```python
from build123d import *

# Parameters (mm, degrees)
SKETCH1_R           = 1.5
SKETCH1_R_2         = 1.375
SKETCH1_R_3         = 1.6
SKETCH1_R_4         = 1.625
SKETCH1_R_5         = 3.5687
SKETCH1_W           = 50
SKETCH1_H           = 41.5
BOSS_EXTRUDE1_DEPTH = 12.7


with BuildPart() as part:
    # Sketch1 → Boss-Extrude1 (new body)
    with BuildSketch(Plane(origin=(0, 0, 0), x_dir=(1, 0, 0), z_dir=(0, 1, 0))):
        with BuildLine():
            Line((175, -200), (175, 200))
            ThreePointArc((175, 200), (0, 265.753645318), (-175, 200))
            Line((-175, 200), (-175, -200))
            ThreePointArc((-175, -200), (-105.083237909, -244.095295142), (-25, -264.575131106))
            ThreePointArc((-25, -264.575131106), (-12.51388125, -265.458853264), (0, -265.753645318))
            ThreePointArc((0, -265.753645318), (12.51388125, -265.458853264), (25, -264.575131106))
            ThreePointArc((25, -264.575131106), (105.083237909, -244.095295142), (175, -200))
        make_face()
        with Locations((-31, -219.575131106)):
            Circle(SKETCH1_R, mode=Mode.SUBTRACT)
        with Locations((31, -219.575131106)):
            Circle(SKETCH1_R, mode=Mode.SUBTRACT)
        with Locations((22.5, -166)):
            Circle(SKETCH1_R_2, mode=Mode.SUBTRACT)
        with Locations((-31, -254.575131106)):
            Circle(SKETCH1_R, mode=Mode.SUBTRACT)
        with Locations((31, -254.575131106)):
            Circle(SKETCH1_R, mode=Mode.SUBTRACT)
        with Locations((-35.5, -166)):
            Circle(SKETCH1_R_2, mode=Mode.SUBTRACT)
        with Locations((22.5, -80)):
            Circle(SKETCH1_R_2, mode=Mode.SUBTRACT)
        with Locations((-35.5, -80)):
            Circle(SKETCH1_R_2, mode=Mode.SUBTRACT)
        with Locations((0, 117.5)):
            Circle(SKETCH1_R_3, mode=Mode.SUBTRACT)
        with Locations((0, 20.9)):
            Circle(SKETCH1_R_3, mode=Mode.SUBTRACT)
        with Locations((-113.22, 20.9)):
            Circle(SKETCH1_R, mode=Mode.SUBTRACT)
        with Locations((-64.22, 20.9)):
            Circle(SKETCH1_R, mode=Mode.SUBTRACT)
        with Locations((-64.22, 69.81)):
            Circle(SKETCH1_R, mode=Mode.SUBTRACT)
        with Locations((-113.22, 69.81)):
            Circle(SKETCH1_R, mode=Mode.SUBTRACT)
        with Locations((64.22, 20.9)):
            Circle(SKETCH1_R, mode=Mode.SUBTRACT)
        with Locations((113.22, 20.9)):
            Circle(SKETCH1_R, mode=Mode.SUBTRACT)
        with Locations((113.22, 69.81)):
            Circle(SKETCH1_R, mode=Mode.SUBTRACT)
        with Locations((64.22, 69.81)):
            Circle(SKETCH1_R, mode=Mode.SUBTRACT)
        with Locations((-141.42, -31.15)):
            Circle(SKETCH1_R_4, mode=Mode.SUBTRACT)
        with Locations((-46.42, -31.15)):
            Circle(SKETCH1_R_4, mode=Mode.SUBTRACT)
        with Locations((-141.42, -156.15)):
            Circle(SKETCH1_R_4, mode=Mode.SUBTRACT)
        with Locations((-46.42, -156.15)):
            Circle(SKETCH1_R_4, mode=Mode.SUBTRACT)
        with Locations((46.42, -156.15)):
            Circle(SKETCH1_R_4, mode=Mode.SUBTRACT)
        with Locations((141.42, -156.15)):
            Circle(SKETCH1_R_4, mode=Mode.SUBTRACT)
        with Locations((46.42, -31.15)):
            Circle(SKETCH1_R_4, mode=Mode.SUBTRACT)
        with Locations((141.42, -31.15)):
            Circle(SKETCH1_R_4, mode=Mode.SUBTRACT)
        with Locations((-159.12, -101.6)):
            Circle(SKETCH1_R_5, mode=Mode.SUBTRACT)
        with Locations((-159.12, -152.4)):
            Circle(SKETCH1_R_5, mode=Mode.SUBTRACT)
        with Locations((-159.12, 152.4)):
            Circle(SKETCH1_R_5, mode=Mode.SUBTRACT)
        with Locations((-159.12, 101.6)):
            Circle(SKETCH1_R_5, mode=Mode.SUBTRACT)
        with Locations((159.12, -152.4)):
            Circle(SKETCH1_R_5, mode=Mode.SUBTRACT)
        with Locations((159.12, -101.6)):
            Circle(SKETCH1_R_5, mode=Mode.SUBTRACT)
        with Locations((159.12, 101.6)):
            Circle(SKETCH1_R_5, mode=Mode.SUBTRACT)
        with Locations((159.12, 152.4)):
            Circle(SKETCH1_R_5, mode=Mode.SUBTRACT)
        with Locations((-159.12, 187.3)):
            Circle(SKETCH1_R_5, mode=Mode.SUBTRACT)
        with Locations((-159.12, 0)):
            Circle(SKETCH1_R_5, mode=Mode.SUBTRACT)
        with Locations((-159.12, -187.3)):
            Circle(SKETCH1_R_5, mode=Mode.SUBTRACT)
        with Locations((159.12, 187.3)):
            Circle(SKETCH1_R_5, mode=Mode.SUBTRACT)
        with Locations((159.12, 0)):
            Circle(SKETCH1_R_5, mode=Mode.SUBTRACT)
        with Locations((159.12, -187.3)):
            Circle(SKETCH1_R_5, mode=Mode.SUBTRACT)
        with Locations((0, -240.325131106)):
            Rectangle(SKETCH1_W, SKETCH1_H, mode=Mode.SUBTRACT)
        with BuildLine():
            Line((-140.07, -12.7), (-127.37, -12.7))
            ThreePointArc((-127.37, -12.7), (-121.02, -19.05), (-127.37, -25.4))
            Line((-127.37, -25.4), (-140.07, -25.4))
            ThreePointArc((-140.07, -25.4), (-146.42, -19.05), (-140.07, -12.7))
        make_face(mode=Mode.SUBTRACT)
        with BuildLine():
            Line((-140.07, 25.4), (-127.37, 25.4))
            ThreePointArc((-127.37, 25.4), (-121.02, 19.05), (-127.37, 12.7))
            Line((-127.37, 12.7), (-140.07, 12.7))
            ThreePointArc((-140.07, 12.7), (-146.42, 19.05), (-140.07, 25.4))
        make_face(mode=Mode.SUBTRACT)
        with BuildLine():
            Line((140.07, 25.4), (127.37, 25.4))
            ThreePointArc((127.37, 25.4), (121.02, 19.05), (127.37, 12.7))
            Line((127.37, 12.7), (140.07, 12.7))
            ThreePointArc((140.07, 12.7), (146.42, 19.05), (140.07, 25.4))
        make_face(mode=Mode.SUBTRACT)
        with BuildLine():
            Line((140.07, -12.7), (127.37, -12.7))
            ThreePointArc((127.37, -12.7), (121.02, -19.05), (127.37, -25.4))
            Line((127.37, -25.4), (140.07, -25.4))
            ThreePointArc((140.07, -25.4), (146.42, -19.05), (140.07, -12.7))
        make_face(mode=Mode.SUBTRACT)
        with BuildLine():
            Line((-140.07, -161.9), (-127.37, -161.9))
            ThreePointArc((-127.37, -161.9), (-121.02, -168.25), (-127.37, -174.6))
            Line((-127.37, -174.6), (-140.07, -174.6))
            ThreePointArc((-140.07, -174.6), (-146.42, -168.25), (-140.07, -161.9))
        make_face(mode=Mode.SUBTRACT)
        with BuildLine():
            Line((127.37, -161.9), (140.07, -161.9))
            ThreePointArc((140.07, -161.9), (146.42, -168.25), (140.07, -174.6))
            Line((140.07, -174.6), (127.37, -174.6))
            ThreePointArc((127.37, -174.6), (121.02, -168.25), (127.37, -161.9))
        make_face(mode=Mode.SUBTRACT)
        with BuildLine():
            Line((-140.07, 174.6), (-127.37, 174.6))
            ThreePointArc((-127.37, 174.6), (-121.02, 168.25), (-127.37, 161.9))
            Line((-127.37, 161.9), (-140.07, 161.9))
            ThreePointArc((-140.07, 161.9), (-146.42, 168.25), (-140.07, 174.6))
        make_face(mode=Mode.SUBTRACT)
        with BuildLine():
            Line((127.37, 174.6), (140.07, 174.6))
            ThreePointArc((140.07, 174.6), (146.42, 168.25), (140.07, 161.9))
            Line((140.07, 161.9), (127.37, 161.9))
            ThreePointArc((127.37, 161.9), (121.02, 168.25), (127.37, 174.6))
        make_face(mode=Mode.SUBTRACT)
    extrude(amount=BOSS_EXTRUDE1_DEPTH)


solid = part.part
```
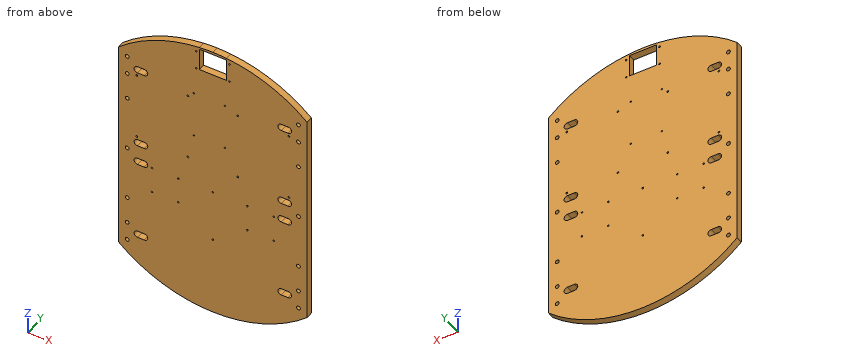
Input: part model. Units: mm. Frame: model coordinates. Round coordinates to 2 decimals unless told otherwise and drop trailing zeros. Loops run counter-clockwise (first coordinate to the right, second up) from the corner with the lowest first, then second, coordinate; pieces in that order, holes last. Notation, with made-up numbers: (62, 64.25) -> (81, 64.25) arc R24 ccw to (81, 93.25) -> close; hole circle Ø3 at (67, 46). An arc over 180 degrees is marked (long way). Write each question's results on one line, items separated by ' | '.
1. Section C-C (x = -94.5). Return loops of the section in (y, z).
Geometry results:
outline: (0, -248.38) -> (12.7, -248.38) -> (12.7, 248.38) -> (0, 248.38) -> close
2. Section A-A (z = 19.05). Return loops of the section in (x, y), and give its area (3 significant figures).
Geometry results:
outline: (-175, 0) -> (-146.42, 0) -> (-146.42, 12.7) -> (-175, 12.7) -> close; (-121.02, 0) -> (121.02, 0) -> (121.02, 12.7) -> (-121.02, 12.7) -> close; (146.42, 0) -> (175, 0) -> (175, 12.7) -> (146.42, 12.7) -> close | area: 3,800 mm2
3. Section B-B (y = 6.75). State how many separate pieces and enclosed holes the cut face has, and give its area (3 significant figures).
Geometry results:
separate pieces: 1 | enclosed holes: 49 | area: 166,000 mm2
4. Ray query, line 1 (X direction, y = 4.75, z = 31.15) (3 decimals); line 2 (X direction, y = 4, z = -69.81); line 3 (X direction, y = 3, z = 101.6). Return the intervals inside material, ascending. Write a range as from..to.
Geometry results:
line 1: -175..-143.045, -139.795..-48.045, -44.795..44.795, 48.045..139.795, 143.045..175 | line 2: -175..-114.72, -111.72..-65.72, -62.72..62.72, 65.72..111.72, 114.72..175 | line 3: -175..-162.69, -155.55..155.55, 162.69..175
5. First-contact query: P1, Ø4, axis at x = -135.5, y = 4, coming from the -Z side; P2, Ø2, axis at x = -51, y = 5, coming from the +Z side; P3, Ø2, axis at x = 38, y = 5.5, coming from the +Z side. Flat tips, straight axial feed; report the tip coordinate or a pass-through.
Geometry results:
P1: z = -229.79 | P2: z = 261.01 | P3: z = 263.17
